Here's how the part is built. I have some questions about the finished solid (model axes, mm). Face numbers are marked on the shaded views. Coordinates: 2 decimals unless noted, no trailing zeros. Write each loop counter-clockwise with the first axis right and the second up, starting at its lowest first coordinate (ties: lowest second). Pieces come first, ordered by that corner, then holes. Notation, with made-up numbers: M -36,14 L -21,14 A30 cw -21,36 Z; hole C 19,66.25 d4. An arc over 180 degrees is marked long. Use a Markdown table: item, result.
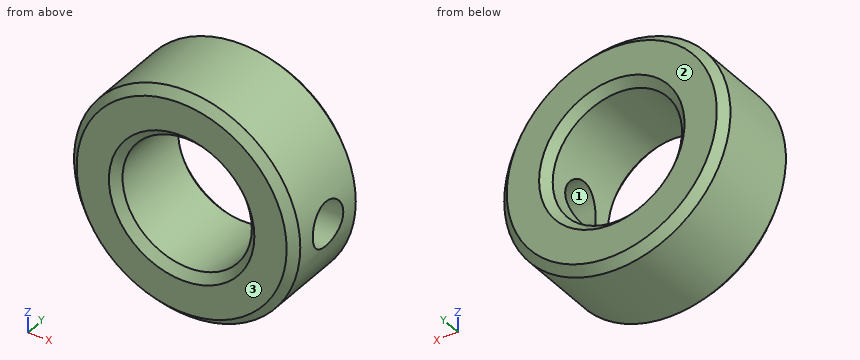
```python
from build123d import *

# Parameters (mm, degrees)
F1_R     = 14
F1_R_2   = 8
F2_DEPTH = 12
F3_SIZE  = 1
F7_D     = 5.5
F7_DEPTH = 14.4
F7_START = 0.2727462
F7_TIP   = 1.6523667023


with BuildPart() as f2:
    # F1 (on Front) → F2 (new body)
    with BuildSketch(Plane.XZ):
        Circle(F1_R)
        Circle(F1_R_2, mode=Mode.SUBTRACT)
    extrude(amount=F2_DEPTH)

    # F3
    f3_edges = [f2.edges().sort_by_distance(p)[0] for p in [
        (14, -6, 0),
        (-14, 0, 0),
        (-14, -12, 0),
        (8, -6, 0),
        (-8, 0, 0),
        (-8, -12, 0),
    ]]
    chamfer(f3_edges, length=F3_SIZE)

    # F7
    # its depths count from where the whole tool has entered the part; down to there all is cleared
    with Locations(Plane.YZ.offset(14).offset(-F7_START)):
        with Locations((-6, 0)):
            Hole(F7_D / 2, depth=F7_DEPTH)
            with Locations((0, 0, -(F7_DEPTH + F7_TIP / 2))):  # 118° drill point
                Cone(0, F7_D / 2, F7_TIP, mode=Mode.SUBTRACT)


solid = f2.part
```
1. We'd pull the mould along Y, two halves only. Please class the marked faces 1, 2 and 3: +Y half, -Y half, draft (parallel to the pull), parting line (faces both ways), or undercut.
Answers follow:
| item | result |
|---|---|
| face 1 | undercut |
| face 2 | +Y half |
| face 3 | -Y half |
2. Will these pins go through, and if not, where does the flat tip stop? pin 1 Ø5 at (y, z) = (-8, 3) entering from +X; pin 2 Ø5 at (x, y) = (-5.5, -9) entering from +Z; pin 3 Ø4 at (y, z) = (-1.5, -1.5) entering from -X; pin 4 Ø1.5 at (y, z) = (-2.5, -4) entering from -X.
Answers follow:
| item | result |
|---|---|
| pin 1 | stops at x = 13.99 |
| pin 2 | stops at z = 13.67 |
| pin 3 | stops at x = -14 |
| pin 4 | stops at x = -13.62 |
3. Suppose I cut it at D-D on y = -6. Write out the boundary of the cut face in (x, z).
Answers follow:
| item | result |
|---|---|
| outline | M 7.51,-2.75 A8 cw long 7.51,2.75 L 13.73,2.75 A14 ccw long 13.73,-2.75 Z |
4. Suppose I cut it at C-C on y = -9.5. Write out the boundary of the cut face in (x, z), and give its area (3 significant figures).
Answers follow:
| item | result |
|---|---|
| outline | C 0,0 d28; hole C 0,0 d16 |
| area | 415 mm2 |
5. I need wall thicknesses on probe 1 along Z at (x, y) = (-0.25, -4.75); probe 2 along Y at (x, z) = (10, 0); probe 3 along Z at (x, y) = (1, -3.75). Which ranges of each line are inside material? Lowest first, please.
Answers follow:
| item | result |
|---|---|
| probe 1 | z = -14 to -8, 8 to 14 |
| probe 2 | y = -12 to -8.75, -3.25 to 0 |
| probe 3 | z = -13.96 to -7.94, 7.94 to 13.96 |
6. Suppose I cut it at B-B on x = 0. Write out the boundary of the cut face in (y, z).
Answers follow:
| item | result |
|---|---|
| outline | M -12,-13 L -11,-14 L -1,-14 L 0,-13 L 0,-9 L -1,-8 L -11,-8 L -12,-9 Z; M -12,9 L -11,8 L -1,8 L 0,9 L 0,13 L -1,14 L -11,14 L -12,13 Z |
7. Suppose I cut it at A-A on z = 0. Write out the boundary of the cut face in (x, y).
Answers follow:
| item | result |
|---|---|
| outline | M -14,-11 L -13,-12 L -9,-12 L -8,-11 L -8,-1 L -9,0 L -13,0 L -14,-1 Z; M 8,-11 L 9,-12 L 13,-12 L 14,-11 L 14,-8.75 L 8,-8.75 Z; M 8,-3.25 L 14,-3.25 L 14,-1 L 13,0 L 9,0 L 8,-1 Z |
